```python
from build123d import *

# Parameters (mm, degrees)
CYLINDER749_R               = 8
CYLINDER749_DEPTH           = 20
CYLINDER749_PLACEMENT_ANGLE = 100
CYLINDER747_R               = 8
CYLINDER747_DEPTH           = 20
CYLINDER747_PLACEMENT_ANGLE = 135
CYLINDER751_R               = 8
CYLINDER751_DEPTH           = 20
CYLINDER753_R               = 8
CYLINDER753_DEPTH           = 20
CYLINDER753_PLACEMENT_ANGLE = 225
CYLINDER746_R               = 8
CYLINDER746_DEPTH           = 20
CYLINDER750_R               = 8
CYLINDER750_DEPTH           = 20
CYLINDER750_PLACEMENT_ANGLE = 55
CYLINDER748_R               = 8
CYLINDER748_DEPTH           = 20
CYLINDER752_R               = 8
CYLINDER752_DEPTH           = 20
CYLINDER752_PLACEMENT_ANGLE = 45
TUBE081_R                   = 38.75
TUBE081_R_2                 = 30
TUBE081_DEPTH               = 8
CHAMFER004_SIZE             = 1


with BuildPart() as obj1:
    # Cylinder749 → Cylinder749 (new body)
    with BuildSketch(Plane.XY):
        Circle(CYLINDER749_R)
    extrude(amount=CYLINDER749_DEPTH)


with BuildPart() as obj1_1:
    # Cylinder749 placement: moved
    add(obj1.part.moved(Location((41.004432, -9.090464, 0))).rotate(Axis((41.004432, -9.090464, 0), (0, 0, 1)), CYLINDER749_PLACEMENT_ANGLE))


with BuildPart() as obj2:
    # Cylinder747 → Cylinder747 (new body)
    with BuildSketch(Plane.XY):
        Circle(CYLINDER747_R)
    extrude(amount=CYLINDER747_DEPTH)


with BuildPart() as obj2_1:
    # Cylinder747 placement: moved
    add(obj2.part.moved(Location((38.80294, 16.072704, 0))).rotate(Axis((38.80294, 16.072704, 0), (0, 0, 1)), CYLINDER747_PLACEMENT_ANGLE))


with BuildPart() as obj3:
    # Cylinder751 → Cylinder751 (new body)
    with BuildSketch(Plane(origin=(16.072704, 38.80294, 0), x_dir=(-1, 0, 0), z_dir=(0, 0, 1))):
        Circle(CYLINDER751_R)
    extrude(amount=CYLINDER751_DEPTH)


with BuildPart() as obj4:
    # Cylinder753 → Cylinder753 (new body)
    with BuildSketch(Plane.XY):
        Circle(CYLINDER753_R)
    extrude(amount=CYLINDER753_DEPTH)


with BuildPart() as obj4_1:
    # Cylinder753 placement: moved
    add(obj4.part.moved(Location((-16.072704, 38.80294, 0))).rotate(Axis((-16.072704, 38.80294, 0), (0, 0, 1)), CYLINDER753_PLACEMENT_ANGLE))


with BuildPart() as obj5:
    # Cylinder746 → Cylinder746 (new body)
    with BuildSketch(Plane(origin=(-38.80294, 16.072704, 0), x_dir=(0, -1, 0), z_dir=(0, 0, 1))):
        Circle(CYLINDER746_R)
    extrude(amount=CYLINDER746_DEPTH)


with BuildPart() as obj6:
    # Cylinder750 → Cylinder750 (new body)
    with BuildSketch(Plane.XY):
        Circle(CYLINDER750_R)
    extrude(amount=CYLINDER750_DEPTH)


with BuildPart() as obj6_1:
    # Cylinder750 placement: moved
    add(obj6.part.moved(Location((-41.004432, -9.090464, 0))).rotate(Axis((-41.004432, -9.090464, 0), (0, 0, -1)), CYLINDER750_PLACEMENT_ANGLE))


with BuildPart() as obj7:
    # Cylinder748 → Cylinder748 (new body)
    with BuildSketch(Plane(origin=(-16.072704, -38.80294, 0), x_dir=(1, 0, 0), z_dir=(0, 0, 1))):
        Circle(CYLINDER748_R)
    extrude(amount=CYLINDER748_DEPTH)


with BuildPart() as compound708:
    # Cylinder752 → Cylinder752 (new body)
    with BuildSketch(Plane.XY):
        Circle(CYLINDER752_R)
    extrude(amount=CYLINDER752_DEPTH)


with BuildPart() as compound708_1:
    # Cylinder752 placement: moved
    add(compound708.part.moved(Location((16.072704, -38.80294, 0))).rotate(Axis((16.072704, -38.80294, 0), (0, 0, 1)), CYLINDER752_PLACEMENT_ANGLE))

    # Compound708: union obj1, obj2, obj3, obj4, obj5, obj6, obj7
    add(obj1_1.part)
    add(obj2_1.part)
    add(obj3.part)
    add(obj4_1.part)
    add(obj5.part)
    add(obj6_1.part)
    add(obj7.part)


with BuildPart() as compound708_2:
    # Compound708 placement: moved
    add(compound708_1.part.moved(Location((0, 0, 56))))


with BuildPart() as chamfer004:
    # Tube081 → Tube081 (new body)
    with BuildSketch(Plane.XY.offset(58)):
        Circle(TUBE081_R)
        Circle(TUBE081_R_2, mode=Mode.SUBTRACT)
    extrude(amount=TUBE081_DEPTH)

    # Cut331: cut Compound708
    add(compound708_2.part, mode=Mode.SUBTRACT)

    # Chamfer004
    chamfer004_edges = [chamfer004.edges().sort_by_distance(p)[0] for p in [
        (38.743471, -0.711323, 66),
        (38.534044, 4.085332, 66),
        (29.684222, -24.90802, 66),
        (0, -38.75, 66),
        (-29.684222, -24.90802, 66),
        (-38.602545, 3.377285, 66),
        (-27.400388, 27.400388, 66),
        (0, 38.75, 66),
        (27.400388, 27.400388, 66),
    ]]
    chamfer(chamfer004_edges, length=CHAMFER004_SIZE)


solid = chamfer004.part
```
Read the model definition and answer for the solid it produces. Units are mm, in the model's axes. Give positions to 0.01 mm unless a question says otherwise; leave off trailing zeros. Write each loop counter-clockwise with the first axis right and the second up, starting at its lowest first coordinate (ties: lowest second). Pieces come first, ordered by that corner, then holes. Notation, with made-up numbers: (-25.75, 86) -> (-0.75, 86) arc R16 cw to (-0.75, 116) -> close; hole circle Ø1 at (64.25, 3). An arc over 180 degrees is marked (long way). Answer in a Markdown table with one row per item.
1) Determine the mould class of faces 1 (the flat face through (11, 28.1, 66)), 2 (the conical face through (27.047, 26.879, 65.618)), 3 (the cylindrical face through (12.9, 31.46, 61.94)) for opening direction X: released by +X, released by -X, zero draft, split by the parting line, or undercut.
Results list:
| item | result |
|---|---|
| face 1 | zero draft |
| face 2 | released by +X |
| face 3 | undercut |
2) Section D-D on x = 15.5 is taken. Give the vertices of the cut face in (y, z).
Results list:
| item | result |
|---|---|
| outline | (-30.82, 58) -> (-25.69, 58) -> (-25.69, 66) -> (-30.82, 66) -> close; (25.69, 58) -> (30.82, 58) -> (30.82, 66) -> (25.69, 66) -> close |
3) Straight lines are drawn through the part: line 1 (Y direction, x = 0, z = 64.75); line 2 (X direction, y = -13, z = 60.75); line 3 (Y direction, x = -27, z = 63.5) (3 decimals). For each, find the intervals that lie inside material, in ascending order. Write a range as [from, to].
Results list:
| item | result |
|---|---|
| line 1 | [-38.75, -30], [30, 38.75] |
| line 2 | [-34.02, -27.04], [27.04, 34.02] |
| line 3 | [-27.795, -13.077], [13.077, 27.795] |
4) This flat-tipped pin is pushed along its axis until it touches: pin 1 Ø4 at (x, z) = (-8, 61.5) entering from +Y. Where does it stop, or does it pass through?
Results list:
| item | result |
|---|---|
| pin 1 | y = 38.28 |
5) Section B-B on z = 59 is taken. Give the vertices of the cut face in (x, y), plus the area to 3 significant figures.
Results list:
| item | result |
|---|---|
| outline | (-38.72, -1.42) arc R8 cw to (-35.7, -15.08) arc R38.75 ccw to (-21.05, -32.54) arc R8 cw to (-8.13, -37.89) arc R38.75 ccw to (8.13, -37.89) arc R8 cw to (21.05, -32.54) arc R38.75 ccw to (35.7, -15.08) arc R8 cw to (38.72, -1.42) arc R38.75 ccw to (37.89, 8.13) arc R8 cw to (32.54, 21.05) arc R38.75 ccw to (21.05, 32.54) arc R8 cw to (8.13, 37.89) arc R38.75 ccw to (-8.13, 37.89) arc R8 cw to (-21.05, 32.54) arc R38.75 ccw to (-32.54, 21.05) arc R8 cw to (-37.89, 8.13) arc R38.75 ccw to start; hole circle Ø60 at (0, 0) |
| area | 1,520 mm^2 |
6) Section A-A on y = 0 is taken. Give the vertices of the cut face in (x, z), plus the area to 3 significant figures.
Results list:
| item | result |
|---|---|
| outline | (-38.75, 58) -> (-30, 58) -> (-30, 66) -> (-37.75, 66) -> (-38.75, 65) -> close; (30, 58) -> (38.75, 58) -> (38.75, 65) -> (37.75, 66) -> (30, 66) -> close |
| area | 139 mm^2 |
